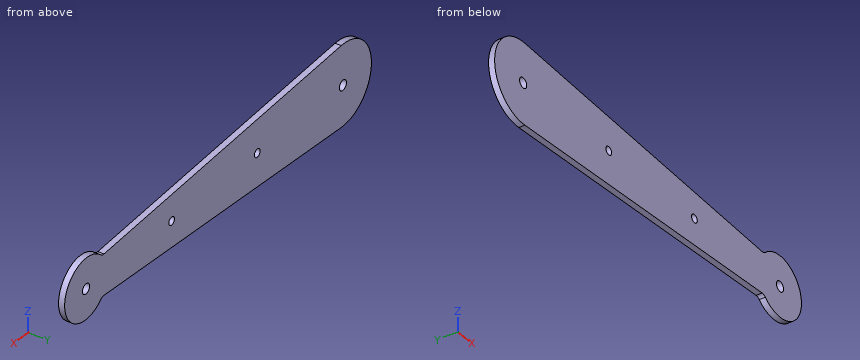
```python
from build123d import *

# Parameters (mm, degrees)
SKETCH1_R           = 2
SKETCH1_R_2         = 2.5
BOSS_EXTRUDE1_DEPTH = 3
FILLET2_R           = 3
FILLET3_R           = 3


with BuildPart() as part:
    # Sketch1 → Boss-Extrude1 (new body)
    with BuildSketch(Plane(origin=(0, 0, 0), x_dir=(1, 0, 0), z_dir=(0, 1, 0))):
        with BuildLine():
            ThreePointArc((1.186783721, 19.964757559), (-20, 0), (1.186783721, -19.964757559))
            Line((1.186783721, -19.964757559), (168.819660113, -10))
            ThreePointArc((168.819660113, -10), (195, 0), (168.819660113, 10))
            Line((168.819660113, 10), (1.186783721, 19.964757559))
        make_face()
        with Locations(Location((60, 0, 0), (0, 0, 270))):
            Circle(SKETCH1_R, mode=Mode.SUBTRACT)
        with Locations(Location((0, 0, 0), (0, 0, 270))):
            Circle(SKETCH1_R_2, mode=Mode.SUBTRACT)
        with Locations(Location((120, 0, 0), (0, 0, 270))):
            Circle(SKETCH1_R, mode=Mode.SUBTRACT)
        with Locations(Location((180, 0, 0), (0, 0, 270))):
            Circle(SKETCH1_R_2, mode=Mode.SUBTRACT)
    extrude(amount=BOSS_EXTRUDE1_DEPTH)

    # Fillet2
    fillet2_edges = [part.edges().sort_by_distance(p)[0] for p in [
        (168.819660113, 1.5, -10),
    ]]
    fillet(fillet2_edges, radius=FILLET2_R)

    # Fillet3
    fillet3_edges = [part.edges().sort_by_distance(p)[0] for p in [
        (168.819660113, 1.5, 10),
    ]]
    fillet(fillet3_edges, radius=FILLET3_R)


solid = part.part
```
Here's how the part is built. I have some questions about the finished solid (model axes, mm). Coordinates: 2 decimals unless noted, no trailing zeros. Loops run counter-clockwise (first coordinate to the right, second up) from the corner with the lowest first, then second, coordinate; pieces in that order, holes last. Notation, with made-up numbers: (-29.5, 60) - (17.5, 60) arc R21 ccw to (17.5, 92) - close; hole circle Ø7 at (24, 36). An arc over 180 degrees is marked (long way). Return JSON: item names as keys, results as strings. Group by question number.
Item 1: If we section it at D-D on x = 120: Write out the boundary of the cut face in (y, z).
Item 2: I need wall thicknesses on line 1 (Z direction, x = 180, y = 1.95); line 2 (X direction, y = 1.35, z = -3.5); line 3 (Z direction, x = 71.5, y = 0.1). Which ranges of each line are inside material? Lowest first, please. Write a range as from..to.
Item 3: If we section it at C-C on y = 2.25: Write out the boundary of the cut face in (x, z).
Item 4: If we section it at B-B on z = 0: Write out the boundary of the cut face in (x, y).
Item 5: If we section it at A-A on x = 180: Write out the boundary of the cut face in (y, z), and give its area (3 significant figures).
Calculated:
{
 "1": {"outline": "(0, -12.9) - (3, -12.9) - (3, -2) - (0, -2) - close; (0, 2) - (3, 2) - (3, 12.9) - (0, 12.9) - close"},
 "2": {"line 1": "z = -15..-2.5, 2.5..15", "line 2": "x = -19.69..194.59", "line 3": "z = -15.79..15.79"},
 "3": {"outline": "(1.19, -19.96) - (167.45, -10.08) arc R3 cw to (169.69, -10.9) arc R15 ccw (long way) to (169.69, 10.9) arc R3 cw to (167.45, 10.08) - (1.19, 19.96) arc R20 ccw (long way) to start; hole circle Ø5 at (0, 0); hole circle Ø4 at (60, 0); hole circle Ø4 at (120, 0); hole circle Ø5 at (180, 0)"},
 "4": {"outline": "(-20, 0) - (-2.5, 0) - (-2.5, 3) - (-20, 3) - close; (2.5, 0) - (58, 0) - (58, 3) - (2.5, 3) - close; (62, 0) - (118, 0) - (118, 3) - (62, 3) - close; (122, 0) - (177.5, 0) - (177.5, 3) - (122, 3) - close; (182.5, 0) - (195, 0) - (195, 3) - (182.5, 3) - close"},
 "5": {"outline": "(0, -15) - (3, -15) - (3, -2.5) - (0, -2.5) - close; (0, 2.5) - (3, 2.5) - (3, 15) - (0, 15) - close", "area": "75.0 mm^2"}
}
